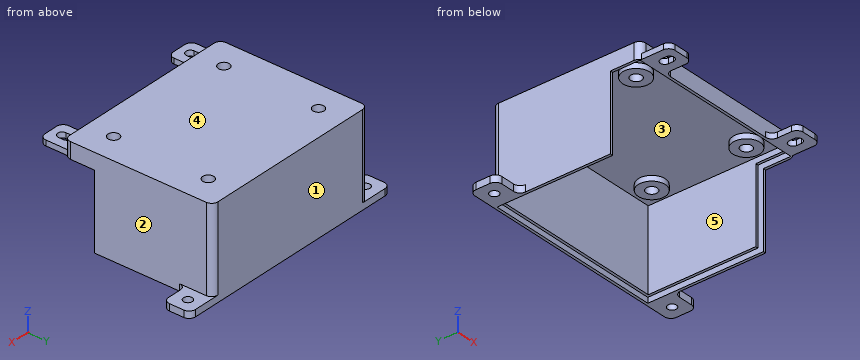
```python
from build123d import *

# Parameters (mm, degrees)
SKETCH1_W           = 82.539998569
SKETCH1_H           = 65.04
BOSS_EXTRUDE1_DEPTH = 43.18
SHELL1_T            = 2.54
CUT_EXTRUDE2_DEPTH  = 124.028758627
SKETCH7_W           = 87.619998569
SKETCH7_H           = 43.18
BOSS_EXTRUDE2_DEPTH = 2.54
CUT_EXTRUDE3_DEPTH  = 2.54
CUT_EXTRUDE4_DEPTH  = 2.54
SKETCH10_W          = 1.27
SKETCH10_H          = 35.56
CUT_EXTRUDE5_DEPTH  = 2.54
SKETCH11_W          = 12.7
SKETCH11_H          = 2.54
BOSS_EXTRUDE3_DEPTH = 12.7
CUT_EXTRUDE7_DEPTH  = 125.717897357
SKETCH13_W          = 12.7
SKETCH13_H          = 12.7
SKETCH13_R          = 2.1
BOSS_EXTRUDE4_DEPTH = 3.175
FILLET2_R           = 3
SKETCH14_R          = 6.35
BOSS_EXTRUDE5_DEPTH = 5
SKETCH15_R          = 2.625
CUT_EXTRUDE8_DEPTH  = 5


with BuildPart() as part:
    # Sketch1 → Boss-Extrude1 (new body)
    with BuildSketch(Plane.XY):
        with Locations((47.599999189, 40.75)):
            Rectangle(SKETCH1_W, SKETCH1_H)
    extrude(amount=BOSS_EXTRUDE1_DEPTH)

    # Shell1
    shell1_openings = [part.faces().sort_by_distance(p)[0] for p in [
        (47.599999189, 73.27, 21.59),
        (47.599999189, 40.75, 0),
    ]]
    offset(amount=SHELL1_T, openings=shell1_openings, kind=Kind.INTERSECTION)

    # Sketch6 → Cut-Extrude2 (cut, through all)
    with BuildSketch(Plane.ZY.offset(-3.789999905)):
        Polygon((2.54, 59.03), (2.54, 73.27), (0, 73.27), (0, 59.03), (0, 3.15), (38.1, 3.15), (38.1, 19.92924), (2.54, 19.92924), align=None)
    extrude(amount=-CUT_EXTRUDE2_DEPTH, mode=Mode.SUBTRACT)

    # Sketch7 → Boss-Extrude2 (add)
    with BuildSketch(Plane(origin=(0, 73.27, 0), x_dir=(1, 0, 0), z_dir=(0, 1, 0))):
        with Locations((47.59999919, -24.13)):
            Rectangle(SKETCH7_W, SKETCH7_H)
    extrude(amount=BOSS_EXTRUDE2_DEPTH)

    # Sketch8 → Cut-Extrude3 (cut)
    with BuildSketch(Plane(origin=(0, 0, 2.54), x_dir=(-1, 0, 0), z_dir=(0, 0, -1))):
        Polygon((-65.405564728, 73.27), (-65.405564728, 74.54), (-90.139998474, 74.54), (-90.139998474, 19.92924), (-88.869998474, 19.92924), (-88.869998474, 73.27), align=None)
        Polygon((-5.059999905, 74.54), (-65.405564728, 74.54), (-65.405564728, 73.27), (-6.329999905, 73.27), (-6.329999905, 19.92924), (-5.059999905, 19.92924), align=None)
    extrude(amount=-CUT_EXTRUDE3_DEPTH, mode=Mode.SUBTRACT)

    # Sketch9 → Cut-Extrude4 (cut)
    with BuildSketch(Plane(origin=(0, 0, 38.1), x_dir=(-1, 0, 0), z_dir=(0, 0, -1))):
        Polygon((-90.139998474, 19.92924), (-90.139998474, 6.96), (-5.059999905, 6.96), (-5.059999905, 19.92924), (-6.329999905, 19.92924), (-6.329999905, 8.23), (-88.869998474, 8.23), (-88.869998474, 19.92924), align=None)
    extrude(amount=-CUT_EXTRUDE4_DEPTH, mode=Mode.SUBTRACT)

    # Sketch10 → Cut-Extrude5 (cut)
    with BuildSketch(Plane.XZ.offset(-19.92924)):
        with Locations((5.694999905, 22.86)):
            Rectangle(SKETCH10_W, SKETCH10_H)
        with Locations((89.504998474, 22.86)):
            Rectangle(SKETCH10_W, SKETCH10_H)
    extrude(amount=-CUT_EXTRUDE5_DEPTH, mode=Mode.SUBTRACT)

    # Sketch11 → Boss-Extrude3 (add)
    with BuildSketch(Plane.XZ.offset(-5.69)):
        with Locations((11.409999905, 39.37)):
            Rectangle(SKETCH11_W, SKETCH11_H)
        with Locations((83.789998474, 39.37)):
            Rectangle(SKETCH11_W, SKETCH11_H)
    extrude(amount=BOSS_EXTRUDE3_DEPTH)

    # Sketch12 → Cut-Extrude7 (cut, through all)
    with BuildSketch(Plane.XY.offset(40.64)):
        with BuildLine():
            Line((9.309999905, 0.61), (9.309999905, -1.683510845))
            ThreePointArc((9.309999905, -1.683510845), (11.409999905, -3.783510845), (13.509999905, -1.683510845))
            Line((13.509999905, -1.683510845), (13.509999905, 0.61))
            ThreePointArc((13.509999905, 0.61), (11.409999905, 2.71), (9.309999905, 0.61))
        make_face()
        with BuildLine():
            Line((81.689998474, 0.61), (81.689998474, -1.683510845))
            ThreePointArc((81.689998474, -1.683510845), (83.789998474, -3.783510845), (85.889998474, -1.683510845))
            Line((85.889998474, -1.683510845), (85.889998474, 0.61))
            ThreePointArc((85.889998474, 0.61), (83.789998474, 2.71), (81.689998474, 0.61))
        make_face()
    extrude(amount=-CUT_EXTRUDE7_DEPTH, mode=Mode.SUBTRACT)

    # Sketch13 → Boss-Extrude4 (add)
    # profile 1 of 2: a face of its own
    with BuildSketch(Plane(origin=(0, 0, 2.54), x_dir=(-1, 0, 0), z_dir=(0, 0, -1))):
        with Locations((-97.759998474, 69.46)):
            Rectangle(SKETCH13_W, SKETCH13_H)
        with Locations((-97.759998474, 69.46)):
            Circle(SKETCH13_R, mode=Mode.SUBTRACT)
    # profile 2 of 2: a face of its own
    with BuildSketch(Plane(origin=(0, 0, 2.54), x_dir=(-1, 0, 0), z_dir=(0, 0, -1))):
        with Locations((2.560000095, 69.46)):
            Rectangle(SKETCH13_W, SKETCH13_H)
        with Locations((2.560000095, 69.46)):
            Circle(SKETCH13_R, mode=Mode.SUBTRACT)
    extrude(amount=-BOSS_EXTRUDE4_DEPTH)

    # Fillet2
    fillet2_edges = [part.edges().sort_by_distance(p)[0] for p in [
        (77.439998474, 5.69, 39.37),
        (77.439998474, -7.01, 39.37),
        (90.139998474, -7.01, 39.37),
        (17.759999905, -7.01, 39.37),
        (5.059999905, -7.01, 39.37),
        (17.759999905, 5.69, 39.37),
        (3.789999905, 63.11, 4.1275),
        (-8.910000095, 63.11, 4.1275),
        (-8.910000095, 75.81, 4.1275),
        (104.109998474, 63.11, 4.1275),
        (91.409998474, 63.11, 4.1275),
        (104.109998474, 75.81, 4.1275),
        (91.409998474, 75.81, 25.7175),
        (3.789999905, 75.81, 25.7175),
        (3.789999905, 5.69, 41.91),
        (91.409998474, 5.69, 41.91),
    ]]
    fillet(fillet2_edges, radius=FILLET2_R)

    # Sketch14 → Boss-Extrude5 (add)
    with BuildSketch(Plane.XY.offset(45.72)):
        with Locations((16.489999905, 63.11)):
            Circle(SKETCH14_R)
        with Locations((16.489999905, 18.39)):
            Circle(SKETCH14_R)
        with Locations((78.709998474, 18.39)):
            Circle(SKETCH14_R)
        with Locations((78.709998474, 63.11)):
            Circle(SKETCH14_R)
    extrude(amount=-BOSS_EXTRUDE5_DEPTH)

    # Sketch15 → Cut-Extrude8 (cut)
    with BuildSketch(Plane.XY.offset(45.72)):
        with Locations((16.489999905, 63.11)):
            Circle(SKETCH15_R)
        with Locations((78.709998474, 63.11)):
            Circle(SKETCH15_R)
        with Locations((16.489999905, 18.39)):
            Circle(SKETCH15_R)
        with Locations((78.709998474, 18.39)):
            Circle(SKETCH15_R)
    extrude(amount=-CUT_EXTRUDE8_DEPTH, mode=Mode.SUBTRACT)


solid = part.part
```
For this review, take the finished solid that the model builds, in its own axes (mm). Face numbers are marked on the shaded views. A direction names the side the tool comes from. Give positions to 0.01 mm unless a question says otherwise; leave off trailing zeros. Write each loop counter-clockwise with the first axis right and the second up, starting at its lowest first coordinate (ties: lowest second). Pieces come first, ordered by that corner, then holes. Notation, with made-up numbers: M -19.75,-39.5 L 14.25,-39.5 A34 ccw 14.25,-1.5 Z; hole C 61,33.25 d9. An arc over 180 degrees is marked long. Answer as a JSON object with one key per item and string values. Group by question number.
Item 1: Consider section B-B on y = 18.39. Write out the cut boundary in (x, z) (3 decimals), plus the area to 3 significant figures.
Item 2: Consider section A-A on x = 11.41. Write out the cut boundary in (y, z).
Item 3: Consider section D-D on z = 22.5. Write out the cut boundary in (x, y).
Item 4: For pin 1 Ø3 at (y, z) = (1, 39.5) entering from -X; pin 2 Ø10 at (x, y) = (19, 61) entering from -Z; pin 3 Ø6 at (x, y) = (54.5, 7) entering from -Z, all flat-tipped, find the tip position at first contact; note any pin that passes through.
Item 5: Tool access review of the marked faces 4 and 5: name each direction out of +Z, -Z, +X, -X, +Y, -Y from which nothing blocks a thin tool from reaching the whole face with its end or side.
Item 6: Draft analysis for pull direction Y (two halves, no side actions). For the marked faces 1, 2 and 3, state which applies: +Y half, -Y half, draft (parallel to the pull), parting line (faces both ways), or undercut.
Item 7: For probe 1 along Y at (x, z) = (16.49, 44.1) (3 decimals); probe 2 along X at (y, z) = (37, 8.5); probe 3 along Y at (x, z) = (16.49, 42.8) (3 decimals), list the stretches that pass through material, from the lowest coordinate up. Write a range as [from, to].
Item 8: Consider section C-C on x = 52. Write out the cut boundary in (y, z).
Check result:
{
 "1": {"outline": "M 3.79,38.1 L 5.06,38.1 L 5.06,40.64 L 6.33,40.64 L 6.33,43.18 L 10.14,43.18 L 10.14,40.72 L 13.865,40.72 L 13.865,45.72 L 3.79,45.72 Z; M 19.115,40.72 L 22.84,40.72 L 22.84,43.18 L 72.36,43.18 L 72.36,40.72 L 76.085,40.72 L 76.085,45.72 L 19.115,45.72 Z; M 81.335,40.72 L 85.06,40.72 L 85.06,43.18 L 88.87,43.18 L 88.87,40.64 L 90.14,40.64 L 90.14,38.1 L 91.41,38.1 L 91.41,45.72 L 81.335,45.72 Z", "area": "252 mm^2"},
 "2": {"outline": "M -7.01,38.1 L -3.78,38.1 L -3.78,40.64 L -7.01,40.64 Z; M 2.71,38.1 L 6.96,38.1 L 6.96,40.64 L 8.23,40.64 L 8.23,43.18 L 14.58,43.18 L 14.58,40.72 L 22.2,40.72 L 22.2,43.18 L 59.3,43.18 L 59.3,40.72 L 66.92,40.72 L 66.92,43.18 L 73.27,43.18 L 73.27,5.08 L 74.54,5.08 L 74.54,2.54 L 75.81,2.54 L 75.81,45.72 L 5.69,45.72 L 5.69,40.64 L 2.71,40.64 Z"},
 "3": {"outline": "M 3.79,19.93 L 5.06,19.93 L 5.06,22.47 L 6.33,22.47 L 6.33,73.27 L 88.87,73.27 L 88.87,22.47 L 90.14,22.47 L 90.14,19.93 L 91.41,19.93 L 91.41,72.81 A3 ccw 88.41,75.81 L 6.79,75.81 A3 ccw 3.79,72.81 Z"},
 "4": {"pin 1": "stops at x = 5.06", "pin 2": "stops at z = 40.72", "pin 3": "stops at z = 38.1"},
 "5": {"face 4": "+Z, +X, -X, +Y, -Y", "face 5": "-Z"},
 "6": {"face 1": "+Y half", "face 2": "draft", "face 3": "undercut"},
 "7": {"probe 1": "y = [5.69, 15.765], [21.015, 60.485], [65.735, 75.81]", "probe 2": "x = [3.79, 6.33], [88.87, 91.41]", "probe 3": "y = [5.69, 8.23], [12.04, 15.765], [21.015, 24.74], [56.76, 60.485], [65.735, 69.46], [73.27, 75.81]"},
 "8": {"outline": "M 5.69,38.1 L 6.96,38.1 L 6.96,40.64 L 8.23,40.64 L 8.23,43.18 L 73.27,43.18 L 73.27,5.08 L 74.54,5.08 L 74.54,2.54 L 75.81,2.54 L 75.81,45.72 L 5.69,45.72 Z"}
}
